```python
from build123d import *

# Parameters (mm, degrees)
EXTRUDE_1_DEPTH = 114.5


with BuildPart() as part:
    # Эскиз1 → Бобышка-Вытянуть1 (new body)
    with BuildSketch(Plane.XY.offset(111.5)):
        with BuildLine():
            Line((9.5, -38.855501541), (9.5, -39.632688529))
            Line((9.5, -39.632688529), (10.5, -39.632688529))
            ThreePointArc((10.5, -39.632688529), (28.991378029, -28.991378029), (39.632688529, -10.5))
            Line((39.632688529, -10.5), (39.632688529, -9.5))
            Line((39.632688529, -9.5), (38.855501541, -9.5))
            ThreePointArc((38.855501541, -9.5), (28.284271247, -28.284271247), (9.5, -38.855501541))
        make_face()
    extrude(amount=-EXTRUDE_1_DEPTH)


solid = part.part
```
CAD build for the part. Positions are in the model's coordinates, mm. Round coordinates to 2 decimals unless told otherwise and drop trailing zeros. Order: outer loops, then holes, each group sorted by start corner. A loop starts at its lowest first (then second) coordinate and runs counter-clockwise, first axis right, second up. Notation, with made-up numbers: (88.25, -22.75) - (103.25, -22.75) arc R18 cw to (103.25, 2.25) - close; hole circle Ø8 at (86, 16). An arc over 180 degrees is marked (long way). Answer as CSV lines item,"result". Start each with the question number.
1. Saw through at A-A, the plane z = 79. Write the cut outline in (x, y), and give its area (3 significant figures).
2. Saw through at B-B, the plane y = -22. Write the cut outline in (x, z).
3. Saw through at C-C, the plane x = 23. Write the cut outline in (y, z), and give its area (3 significant figures).
4. Drill centre lines: L1, parallel to Y at x = 19, z = 61; L2, parallel to X at y = -13, z = 47.5; L3, parallel to Y at x = 33, z = 7. Where is each one in solid material? Low to high. Write a range as [from, to].
5. Pin check, flat tips, straight feed: pin 1 (6 mm diameter, centred on y = -26, z = 52, fed in from -X); pin 2 (8 mm diameter, centred on x = 29, z = 34, fed in from -Y); pin 3 (5 mm diameter, centred on x = 27, z = 51, fed in from +Y); pin 4 (5 mm diameter, centred on x = 27, y = -36, fed in from +Z). Stop position of each tip, or through.
Model answer:
1,outline,"(9.5, -39.63) - (10.5, -39.63) arc R41 ccw to (39.63, -10.5) - (39.63, -9.5) - (38.86, -9.5) arc R40 cw to (9.5, -38.86) - close"
1,area,"44.2 mm²"
2,outline,"(33.41, -3) - (34.6, -3) - (34.6, 111.5) - (33.41, 111.5) - close"
3,outline,"(-33.94, -3) - (-32.73, -3) - (-32.73, 111.5) - (-33.94, 111.5) - close"
3,area,"139 mm²"
4,L1,"y = [-36.33, -35.2]"
4,L2,"x = [37.83, 38.88]"
4,L3,"y = [-24.33, -22.61]"
5,pin 1,"stops at x = 27.55"
5,pin 2,"stops at y = -32.5"
5,pin 3,"stops at y = -27.01"
5,pin 4,"passes through"
